Geometry: final body of the model. Coordinates: model frame, mm. A direction names the side the tool comes from. Give positions to 0.01 mm unless a question says otherwise; leave off trailing zeros. Write each loop counter-clockwise with the first axis right and the second up, starting at its lowest first coordinate (ties: lowest second). Pieces come first, ordered by that corner, then holes. Notation, with made-up numbers: M 46.5,62.25 L 51.5,62.25 A8 ccw 51.5,71.25 Z; hole C -12,13.5 d6. An arc over 180 degrees is marked long. Use a Markdown table: item, result. Add a question column.
1) Section D-D on x = 162. Return the cut outline in (y, z), then the cut area to 3 significant figures.
2) Section C-C on y = -40. Return the cut outline in (x, z), then the cut area to 3 significant figures.
3) Draft query along Y for faces 1 (the cylindrical face through (-43.36, 104.81, 1.97)), 2 (the flat face through (-113, 1, 4)), 3 (the flat face through (-230.26, 2.93, 1.97)), 4 (the flat face through (-305.022, -57.556, 1.972)). Return one class per face: +Y half, -Y half, draft (parallel to the pull), parting line (faces both ways), or undercut.
4) Section A-A on z = 3. Return the cut outline in (x, y).
5) Line query: line 1 (Y direction, x = -155.5, z = 0.75); line 2 (Y direction, x = -107.5, z = 2); line 3 (X direction, y = -72.5, z = 3.65). Output: solid intervals per line, ascending.
6) Set-up query: faces 5 (the flat face through (-113, 1, 0)), 6 (the flat face through (-220.41, -2.93, 1.97)), 7 (the flat face through (-122.946, 47.565, 1.972)). Return all of +Z, -Z, +X, -X, +Y, -Y with unobstructed straight access to the full face (end or side cutting, diameter ignored); none if empty.
7) Section B-B on x = -246. Return the cut outline in (y, z), then the cut area to 3 significant figures.
8) Pin query (flat end, axial travel): pin 1 (1.5 mm diameter, centred on x = 15.5, z = 0.5, fed in from +Y); pin 2 (2 mm diameter, centred on x = -31.5, z = 1.5, fed in from -Y); pin 3 (2 mm diameter, centred on x = -79.5, z = 3, fed in from +Y). Return the tip coordinate at first contact, or that it passes through.
```python
from build123d import *

# Parameters (mm, degrees)
EXTRUDE_1_DEPTH = 4


with BuildPart() as part:
    # 草图1 → 凸台-拉伸1 (new body)
    with BuildSketch(Plane.XY):
        with BuildLine():
            Line((-196.671823256, 5), (-47.126996537, 91.339745962))
            ThreePointArc((-47.126996537, 91.339745962), (-43.466742499, 105), (-57.126996537, 108.660254038))
            Line((-57.126996537, 108.660254038), (-403.537158051, -91.339745962))
            ThreePointArc((-403.537158051, -91.339745962), (-407.197412089, -105), (-393.537158051, -108.660254038))
            Line((-393.537158051, -108.660254038), (-213.992331332, -5))
            Line((-213.992331332, -5), (84.039471365, -5))
            Line((84.039471365, -5), (162.432840625, -5))
            Line((162.432840625, -5), (232.716639262, -5))
            Line((232.716639262, -5), (232.716639262, 5))
            Line((232.716639262, 5), (162.432840625, 5))
            Line((162.432840625, 5), (84.039471365, 5))
            Line((84.039471365, 5), (-196.671823256, 5))
        make_face()
        with BuildLine():
            Line((-401.037158051, -95.669872981), (-54.626996537, 104.330127019))
            ThreePointArc((-54.626996537, 104.330127019), (-47.796869518, 102.5), (-49.626996537, 95.669872981))
            Line((-49.626996537, 95.669872981), (-396.037158051, -104.330127019))
            ThreePointArc((-396.037158051, -104.330127019), (-402.86728507, -102.5), (-401.037158051, -95.669872981))
        make_face(mode=Mode.SUBTRACT)
    extrude(amount=EXTRUDE_1_DEPTH)


solid = part.part
```
Found:
| question | item | result |
|---|---|---|
| 1 | outline | M -5,0 L 5,0 L 5,4 L -5,4 Z |
| 1 | area | 40.0 mm² |
| 2 | outline | M -314.61,0 L -304.61,0 L -304.61,4 L -314.61,4 Z; M -284.61,0 L -274.61,0 L -274.61,4 L -284.61,4 Z |
| 2 | area | 80.0 mm² |
| 3 | face 1 | undercut |
| 3 | face 2 | draft |
| 3 | face 3 | undercut |
| 3 | face 4 | -Y half |
| 4 | outline | M -403.54,-91.34 A10 ccw -393.54,-108.66 L -213.99,-5 L 232.72,-5 L 232.72,5 L -196.67,5 L -47.13,91.34 A10 ccw -57.13,108.66 Z; hole M -401.04,-95.67 A5 ccw -396.04,-104.33 L -49.63,95.67 A5 ccw -54.63,104.33 Z |
| 5 | line 1 | -5 to 5, 28.77 to 34.54, 46.09 to 51.86 |
| 5 | line 2 | -5 to 5, 56.48 to 62.26, 73.8 to 79.58 |
| 5 | line 3 | -370.91 to -360.91, -340.91 to -330.91 |
| 6 | face 5 | -Z, +X, -X, +Y, -Y |
| 6 | face 6 | +Z, -Z |
| 6 | face 7 | +Z, -Z, +X |
| 7 | outline | M -23.48,0 L -17.71,0 L -17.71,4 L -23.48,4 Z; M -6.16,0 L -0.39,0 L -0.39,4 L -6.16,4 Z |
| 7 | area | 46.2 mm² |
| 8 | pin 1 | y = 5 |
| 8 | pin 2 | y = -5 |
| 8 | pin 3 | y = 96.32 |
